Source: CAD feature listing. Evaluate the final solid. Frame: model axes, mm. Face numbers are marked on the shaded views. A direction names the side the tool comes from. Give positions to 0.01 mm unless a question says otherwise; leave off trailing zeros. Order: outer loops, then holes, each group sorted by start corner. A loop starts at its lowest first (then second) coordinate and runs counter-clockwise, first axis right, second up. Notation, with made-up numbers: (81.25, 79.5) - (123.25, 79.5) arc R5 cw to (123.25, 86.5) - close; hole circle Ø7 at (63, 33.25). An arc over 180 degrees is marked (long way). Use CSV: the item, a comma, the result in double quotes.
```python
from build123d import *

# Parameters (mm, degrees)
F0_R      = 30
F1_DEPTH  = 15
F2_R      = 15.05
F3_DEPTH  = 5
F4_DEPTH  = 6
F5_R      = 20
F6_DEPTH  = 15
F7_R      = 30
F7_R_2    = 20
F8_DEPTH  = 15
F9_W      = 12.9903810568
F9_H      = 30
F10_DEPTH = 10.1
F11_R     = 3.2
F12_DEPTH = 25.98076
F13_R     = 8.45
F14_DEPTH = 25


with BuildPart() as f1:
    # F0 (on Top) → F1 (new body)
    with BuildSketch(Plane.XY):
        Circle(F0_R)
    extrude(amount=F1_DEPTH)

    # F2 (on face) → F3 (cut)
    with BuildSketch(Plane.XY.offset(15)):
        Circle(F2_R)
    extrude(amount=-F3_DEPTH, mode=Mode.SUBTRACT)

    # F4 (add): a face of the model
    f4_faces = [f1.faces().sort_by_distance(p)[0] for p in [
        (-29.1514718626, 0, 15),
    ]]
    extrude(f4_faces, amount=F4_DEPTH)

    # F5 (on face) → F6 (join)
    with BuildSketch(Plane(origin=(0, 0, 0), x_dir=(1, 0, 0), z_dir=(0, 0, -1))):
        Circle(F5_R)
    extrude(amount=F6_DEPTH)

    # F7 (on face) → F8 (join)
    with BuildSketch(Plane(origin=(0, 0, -15), x_dir=(1, 0, 0), z_dir=(0, 0, -1))):
        Circle(F7_R)
        Circle(F7_R_2, mode=Mode.SUBTRACT)
        Circle(F7_R_2)
    extrude(amount=F8_DEPTH)

    # F9 (on face) → F10 (join)
    with BuildSketch(Plane(origin=(0, 0, -30), x_dir=(1, 0, 0), z_dir=(0, 0, -1))):
        with Locations((6.4951905284, 0)):
            Rectangle(F9_W, F9_H)
        with Locations((19.4855715851, 0)):
            Rectangle(F9_W, F9_H)
    extrude(amount=F10_DEPTH)

    # F11 (on face) → F12 (join)
    with BuildSketch(Plane.YZ.offset(25.9807621135)):
        with BuildLine():
            Line((15, -40.1), (0, -40.1))
            Line((0, -40.1), (-15, -40.1))
            ThreePointArc((-15, -40.1), (-6.688399949, -71.0645284311), (19.5714285714, -52.6714285714))
            ThreePointArc((19.5714285714, -52.6714285714), (18.3930998597, -45.9830286224), (15, -40.1))
        make_face()
        with Locations((0, -52.6714285714)):
            Circle(F11_R, mode=Mode.SUBTRACT)
    extrude(amount=-F12_DEPTH)

    # F13 (on face) → F14 (join)
    with BuildSketch(Plane.XY.offset(10)):
        Circle(F13_R)
    extrude(amount=F14_DEPTH)


solid = f1.part
```
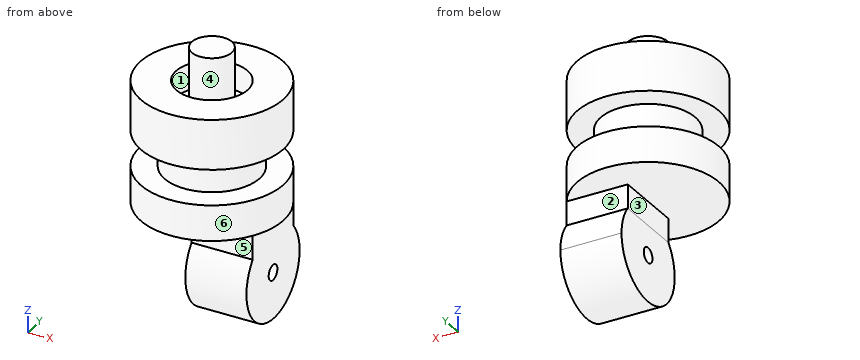
Item 1: Mould query, pull axis Y, two halves, no side actions, for the marked faces 4, 5 and 6. Classes: released by +Y, released by -Y, zero draft, split by the parting line, or undercut.
Filled in:
face 4,"undercut"
face 5,"released by -Y"
face 6,"split by the parting line"
Item 2: Section C-C on x = 4.5. Return the cut outline in (y, z).
Filled in:
outline,"(-29.66, -30) - (-15, -30) - (-15, -40.1) arc R19.57 ccw (long way) to (15, -40.1) - (15, -30) - (29.66, -30) - (29.66, -15) - (19.49, -15) - (19.49, 0) - (29.66, 0) - (29.66, 21) - (14.36, 21) - (14.36, 10) - (7.15, 10) - (7.15, 35) - (-7.15, 35) - (-7.15, 10) - (-14.36, 10) - (-14.36, 21) - (-29.66, 21) - (-29.66, 0) - (-19.49, 0) - (-19.49, -15) - (-29.66, -15) - close; hole circle Ø6.4 at (0, -52.67)"
Item 3: Set-up query: the marked faces 1, 2 and 3. Return all of +Z, -Z, +X, -X, +Y, -Y with unobstructed straight access to the full face (end or side cutting, diameter ignored); none if empty.
Filled in:
face 1,"+Z"
face 2,"+X, -X, +Y"
face 3,"-Z, -X, +Y, -Y"
Item 4: Material intervals for line 1 (Y direction, x = 0, z = 15); line 2 (Z direction, x = -16, y = -25); line 3 (Z direction, x = 16.75, y = 0), sorted ascending. Write a range as from..to.
Filled in:
line 1,"y = -30..-15.05, -8.45..8.45, 15.05..30"
line 2,"z = -30..-15, 0..21"
line 3,"z = -72.24..-55.87, -49.47..21"
Item 5: Section D-D on z = -36.5. Return the cut outline in (x, y), then the cut area to 3 significant figures.
Filled in:
outline,"(0, -15) - (25.98, -15) - (25.98, 15) - (0, 15) - close"
area,"779 mm2"
Item 6: Section B-B on x = 23. Return the cut outline in (y, z).
Filled in:
outline,"(-19.26, -30) - (-15, -30) - (-15, -40.1) arc R19.57 ccw (long way) to (15, -40.1) - (15, -30) - (19.26, -30) - (19.26, -15) - (-19.26, -15) - close; (-19.26, 0) - (19.26, 0) - (19.26, 21) - (-19.26, 21) - close; hole circle Ø6.4 at (0, -52.67)"
Item 7: First-contact query: pin 1 (2 mm diameter, centred on x = 6, y = -8.5, fed in from -Z); pin 2 (1.5 mm diameter, centred on x = 3.5, y = 21, fed in from +Z); pin 3 (6 mm diameter, centred on x = 19.5, z = -10.5, fed in from -Y). Flat tips, straight axial feed; report the tip coordinate or a pass-through.
Filled in:
pin 1,"stops at z = -70.75"
pin 2,"stops at z = 21"
pin 3,"stops at y = -11.3"
